Work out the finished part from the listing and answer in its coordinate system (mm). Coordinates: 2 decimals unless noted, no trailing zeros. Order: outer loops, then holes, each group sorted by start corner. A loop starts at its lowest first (then second) coordinate and runs counter-clockwise, first axis right, second up. Notation, with made-up numbers: (57, -37.5) -> (111, -37.5) arc R20 cw to (111, -32.5) -> close; hole circle Ø7 at (50.25, 42.25). An arc over 180 degrees is marked (long way). Write item = value, one per line. Start each with the question number.
Q1. For a pull along X with two mould halves and no side action, classify faces 1 (the flat face through (-76.414, -1, -5)), 2 (the cylindrical face through (46.548, 9.412, -4.508)), 3 (the flat face through (-1, 1, -9.144)) as +X half, -X half, draft (parallel to the pull), parting line (faces both ways), or undercut.
Q2. The part is cut by section A-A, the plane x = 39.5. Determine the outline of the cut face in (y, z).
Q3. The part is cut by section B-B, the plane y = 20. Determine the outline of the cut face in (x, z).
Q4. Straight lines are drawn through the part: L1, parallel to X at y = 18.5, z = -4.5; L2, parallel to Y at x = 44, z = -2.5; L3, parallel to X at y = 22, z = -4. For each, find the intervals that lie inside material, in ascending order. Write a range as from..to.
```python
from build123d import *

# Parameters (mm, degrees)
SKETCH1_W      = 152.828642472
SKETCH1_H      = 152.828642472
SKETCH1_R      = 9.347426307
EXTRUDE1_DEPTH = 9.144


with BuildPart() as part:
    # Sketch1 → Extrude1 (new body)
    with BuildSketch(Plane.XY):
        Rectangle(SKETCH1_W, SKETCH1_H)
        with Locations((42.234252899, 17.704783599)):
            Circle(SKETCH1_R, mode=Mode.SUBTRACT)
    extrude(amount=-EXTRUDE1_DEPTH)


solid = part.part
```
Model answer:
q1.face_1 = -X half
q1.face_2 = undercut
q1.face_3 = draft
q2.outline = (-76.41, -9.14) -> (8.77, -9.14) -> (8.77, 0) -> (-76.41, 0) -> close; (26.64, -9.14) -> (76.41, -9.14) -> (76.41, 0) -> (26.64, 0) -> close
q3.outline = (-76.41, -9.14) -> (33.17, -9.14) -> (33.17, 0) -> (-76.41, 0) -> close; (51.3, -9.14) -> (76.41, -9.14) -> (76.41, 0) -> (51.3, 0) -> close
q4.L1 = -76.41..32.92, 51.55..76.41
q4.L2 = -76.41..8.53, 26.88..76.41
q4.L3 = -76.41..33.93, 50.54..76.41
